Source: CAD feature listing. Evaluate the final solid. Frame: model axes, mm. Coordinates: 2 decimals unless noted, no trailing zeros. Order: outer loops, then holes, each group sorted by start corner. A loop starts at its lowest first (then second) coordinate and runs counter-clockwise, first axis right, second up.
```python
from build123d import *

# Parameters (mm, degrees)
BOSS_EXTRUDE1_DEPTH = 1.5875
SKETCH2_W           = 88.9
SKETCH2_H           = 342.9
CUT_EXTRUDE1_DEPTH  = 2.5875
SKETCH4_W           = 1292.225
SKETCH4_H           = 800.002961837
CUT_EXTRUDE2_DEPTH  = 2.5875
CUT_EXTRUDE3_DEPTH  = 2.5875
FILLET1_R           = 3.175
FILLET2_R           = 6.35


with BuildPart() as part:
    # Sketch1 → Boss-Extrude1 (new body)
    with BuildSketch(Plane.XY):
        with BuildLine():
            Line((1292.225, 0), (-1292.225, 0))
            Line((-1292.225, 0), (-304.303617208, 800.002961837))
            ThreePointArc((-304.303617208, 800.002961837), (0, 573.0875), (304.303617208, 800.002961837))
            Line((304.303617208, 800.002961837), (1292.225, 0))
        make_face()
    extrude(amount=BOSS_EXTRUDE1_DEPTH)

    # Sketch2 → Cut-Extrude1 (cut, through all)
    with BuildSketch(Plane.XY.offset(1.5875)):
        with Locations((0, 171.45)):
            Rectangle(SKETCH2_W, SKETCH2_H)
    extrude(amount=-CUT_EXTRUDE1_DEPTH, mode=Mode.SUBTRACT)

    # Sketch4 → Cut-Extrude2 (cut, through all)
    with BuildSketch(Plane.XY.offset(1.5875)):
        with Locations((646.1125, 400.001480919)):
            Rectangle(SKETCH4_W, SKETCH4_H)
    extrude(amount=-CUT_EXTRUDE2_DEPTH, mode=Mode.SUBTRACT)

    # Sketch5 → Cut-Extrude3 (cut, through all)
    with BuildSketch(Plane.XY.offset(1.5875)):
        Polygon((-44.45, 253.902961837), (-978.680954392, 253.902961837), (-1292.225, 0), (-44.45, 0), align=None)
    extrude(amount=-CUT_EXTRUDE3_DEPTH, mode=Mode.SUBTRACT)

    # Fillet1
    fillet1_edges = [part.edges().sort_by_distance(p)[0] for p in [
        (-44.45, 342.9, 0.79375),
        (0, 342.9, 0.79375),
        (0, 573.0875, 0.79375),
        (-44.45, 253.902961837, 0.79375),
        (-304.303617208, 800.002961837, 0.79375),
    ]]
    fillet(fillet1_edges, radius=FILLET1_R)

    # Fillet2
    fillet2_edges = [part.edges().sort_by_distance(p)[0] for p in [
        (-978.680954392, 253.902961837, 0.79375),
    ]]
    fillet(fillet2_edges, radius=FILLET2_R)


solid = part.part
```
Q1. Section query B-B on x = -148.5. Output: boundary loops of the cut face in (y, z), plus the area to 3 significant figures.
Solutions:
outline: (253.9, 0) - (609.96, 0) - (609.96, 1.59) - (253.9, 1.59) - close
area: 565 mm2
Q2. Pin query (flat end, axial travel): P1, Ø0.8, axis at y = 311, z = 0.5, coming from the +X side. Return the tip coordinate at first contact, or that it passes through.
Solutions:
P1: stops at x = -44.45
Q3. Section query C-C on y = 329.5. Output: boundary loops of the cut face in (x, z).
Solutions:
outline: (-885.33, 0) - (-44.45, 0) - (-44.45, 1.59) - (-885.33, 1.59) - close
Q4. Material intervals for line 1 along Y through (x, z) = (-433, 1); line 2 along Y through (x, z) = (-335.5, 0.65); line 3 along X through (y, z) = (366.5, 0.2), sorted ascending.
Solutions:
line 1: y = 253.9 to 695.79
line 2: y = 253.9 to 774.74
line 3: x = -839.64 to 0
